Work out the finished part from the listing and answer in its coordinate system (mm). Face numbers are marked on the shaded views. A direction names the side the tool comes from. Round coordinates to 2 decimals unless told otherwise and drop trailing zeros. Write each loop counter-clockwise with the first axis right and the second up, starting at its lowest first coordinate (ties: lowest second). Pieces come first, ordered by that corner, then holes. Notation, with made-up numbers: M 39,34 L 95,34 A38 cw 95,72 Z; hole C 35.25,78.25 d6. An arc over 180 degrees is marked long. One line per item, written item: value. Start each with the question number.
Q1. Find section A-A (z = 19.15). Write down the section's boundary in (x, y), and give its area (3 significant figures).
Q2. A tool of negligible diameter and unlimited length cuts with its end or side. For the marked faces 1 and 2, from which of +Z, -Z, +X, -X, +Y, -Y can it reach the whole face along a straight path? Write none if from no direction.
Q3. Find section B-B (x = 8.5). Write down the section's boundary in (y, z), and give its area (3 significant figures).
Q4. The mould has two halves that part along X. Classify the marked faces 3, 4, 5 and 6: released by +X, released by -X, zero draft, split by the parting line, or undercut.
Q5. Consider probe 1 along Y at (x, z) = (10.75, 21.05); probe 2 along X at (y, z) = (-19, 19.85); probe 3 along Z at (x, y) = (13.75, -18.25). Determine where each line is inside the solid, lowest interval first.
Q6. Find section C-C (x = 20.25). Write down the section's boundary in (y, z), and give its area (3 significant figures).
Q7. Given pin 1 Ø3 at (x, y) = (10, -19) entering from +Z, flat-ended and moving along its own axis, determine where the tip first touches the part or whether it passes through.
from build123d import *

# Parameters (mm, degrees)
CROQUIS1_W                        = 21.8
CROQUIS1_H                        = 30
SALIENTE_EXTRUIR1_DEPTH           = 21.8
CROQUIS6_R                        = 2
CORTAR_EXTRUIR2_DEPTH             = 21.8
CORTAR_EXTRUIR4_REACH             = 45.017
CROQUIS11_R                       = 3.5
CROQUIS11_W                       = 3.4
CROQUIS11_H                       = 8.4
CORTAR_EXTRUIR4_DIRECTION_2_DEPTH = 3.5
REDONDEO1_R                       = 5
CROQUIS13_R                       = 3.5
CORTAR_EXTRUIR6_DEPTH             = 3.5
CROQUIS16_W                       = 10.1
CROQUIS16_H                       = 20.1
CORTAR_EXTRUIR7_DEPTH             = 2
CROQUIS17_W                       = 10.1
CROQUIS17_H                       = 20.1
CORTAR_EXTRUIR8_DEPTH             = 2.1
CORTAR_EXTRUIR9_START             = -3.5
CROQUIS7_R                        = 3.5
CORTAR_EXTRUIR9_DEPTH             = 3.5
CORTAR_EXTRUIR10_REACH            = 45.017
CROQUIS18_W                       = 18.8
CROQUIS18_H                       = 30


with BuildPart() as part:
    # Croquis1 → Saliente-Extruir1 (new body)
    with BuildSketch(Plane(origin=(0, 0, 0), x_dir=(0, 0, -1), z_dir=(1, 0, 0))):
        with Locations((-10.9, -15)):
            Rectangle(CROQUIS1_W, CROQUIS1_H)
    extrude(amount=SALIENTE_EXTRUIR1_DEPTH)

    # Croquis6 → Cortar-Extruir2 (cut)
    with BuildSketch(Plane.ZY):
        with Locations((10.9, -22)):
            Circle(CROQUIS6_R)
        with Locations((10.9, -7)):
            Circle(CROQUIS6_R)
    extrude(amount=-CORTAR_EXTRUIR2_DEPTH, mode=Mode.SUBTRACT)

    # Cortar-Extruir4: up to this face of the body (flat: up to its plane)
    cortar_extruir4_end = Plane(part.part.faces().sort_by_distance((10.9, 0, 10.9))[0])
    # Croquis11 → Cortar-Extruir4 (cut, up to the picked face)
    with BuildSketch(Plane.XZ.offset(30), mode=Mode.PRIVATE) as cortar_extruir4_sk1:
        with Locations(Location((13.4, 10.9, 0), (0, 0, 270))):
            Circle(CROQUIS11_R)
    cortar_extruir4_tool1 = split(extrude(cortar_extruir4_sk1.sketch, amount=-CORTAR_EXTRUIR4_REACH, mode=Mode.PRIVATE), bisect_by=cortar_extruir4_end, keep=Keep.BOTH, mode=Mode.PRIVATE)
    # Croquis11 → Cortar-Extruir4 (cut, up to the picked face)
    with BuildSketch(Plane.XZ.offset(30), mode=Mode.PRIVATE) as cortar_extruir4_sk2:
        with Locations((7.2, 10.9)):
            Rectangle(CROQUIS11_W, CROQUIS11_H)
    cortar_extruir4_tool2 = split(extrude(cortar_extruir4_sk2.sketch, amount=-CORTAR_EXTRUIR4_REACH, mode=Mode.PRIVATE), bisect_by=cortar_extruir4_end, keep=Keep.BOTH, mode=Mode.PRIVATE)
    add(cortar_extruir4_tool1.solids().sort_by(Axis((13.4, -30, 10.9), (0, 1, 0)))[0], mode=Mode.SUBTRACT)
    add(cortar_extruir4_tool2.solids().sort_by(Axis((7.2, -30, 10.9), (0, 1, 0)))[0], mode=Mode.SUBTRACT)

    # Croquis11 → Cortar-Extruir4 direction 2 (cut)
    with BuildSketch(Plane.XZ.offset(30)):
        with Locations(Location((13.4, 10.9, 0), (0, 0, 270))):
            Circle(CROQUIS11_R)
        with Locations((7.2, 10.9)):
            Rectangle(CROQUIS11_W, CROQUIS11_H)
    extrude(amount=CORTAR_EXTRUIR4_DIRECTION_2_DEPTH, mode=Mode.SUBTRACT)

    # Redondeo1
    # the kernel refuses this fillet: 5 mm, written as the material it takes off along each edge
    with BuildSketch(Plane(origin=(21.8, -30, 34.3), x_dir=(0, 1, 0), z_dir=(0, 0, -1)), Plane(origin=(0, 0, -12.5), x_dir=(1, 0, 0), z_dir=(0, 0, 1))) as redondeo1_piece_1:
        with BuildLine():
            CenterArc((REDONDEO1_R, -REDONDEO1_R), REDONDEO1_R, 90, 90)
            Line((0, -REDONDEO1_R), (0, 0))
            Line((0, 0), (REDONDEO1_R, 0))
        make_face()
    extrude(amount=46.8, mode=Mode.SUBTRACT)
    with BuildSketch(Plane(origin=(21.8, 0, -12.5), x_dir=(-1, 0, 0), z_dir=(0, 0, 1)), Plane(origin=(0, -30, 34.3), x_dir=(0, 1, 0), z_dir=(0, 0, -1))) as redondeo1_piece_2:
        with BuildLine():
            CenterArc((REDONDEO1_R, REDONDEO1_R), REDONDEO1_R, 180, 90)
            Line((0, REDONDEO1_R), (0, 0))
            Line((0, 0), (REDONDEO1_R, 0))
        make_face()
    extrude(amount=46.8, mode=Mode.SUBTRACT)

    # Croquis13 → Cortar-Extruir6 (cut)
    with BuildSketch(Plane.ZY):
        with Locations((10.9, -7)):
            Circle(CROQUIS13_R)
        with Locations(Location((10.9, -22, 0), (0, 0, 301.002719134))):
            Circle(CROQUIS13_R)
    extrude(amount=-CORTAR_EXTRUIR6_DEPTH, mode=Mode.SUBTRACT)

    # Croquis16 → Cortar-Extruir7 (cut)
    with BuildSketch(Plane.XY.offset(21.8)):
        with Locations((10.9, -15)):
            Rectangle(CROQUIS16_W, CROQUIS16_H)
    extrude(amount=-CORTAR_EXTRUIR7_DEPTH, mode=Mode.SUBTRACT)

    # Croquis17 → Cortar-Extruir8 (cut)
    with BuildSketch(Plane(origin=(0, 0, 0), x_dir=(-1, 0, 0), z_dir=(0, 0, -1))):
        with Locations((-10.9, -15)):
            Rectangle(CROQUIS17_W, CROQUIS17_H)
    extrude(amount=-CORTAR_EXTRUIR8_DEPTH, mode=Mode.SUBTRACT)

    # Croquis7 → Cortar-Extruir9 (cut)
    with BuildSketch(Plane(origin=(21.8, 0, 0), x_dir=(0, 0, -1), z_dir=(1, 0, 0)).offset(CORTAR_EXTRUIR9_START)):
        with Locations(Location((-10.9, -22, 0), (0, 0, 238.997280866))):
            Circle(CROQUIS7_R)
        with Locations(Location((-10.9, -7, 0), (0, 0, 180))):
            Circle(CROQUIS7_R)
    extrude(amount=CORTAR_EXTRUIR9_DEPTH, mode=Mode.SUBTRACT)

    # Cortar-Extruir10: up to this face of the body (flat: up to its plane)
    cortar_extruir10_end = Plane(part.part.faces().sort_by_distance((21.8, -14.963855914, 10.9))[0])
    # Croquis18 → Cortar-Extruir10 (cut, up to the picked face)
    with BuildSketch(Plane.ZY, mode=Mode.PRIVATE) as cortar_extruir10_sk1:
        with Locations((9.4, -15)):
            Rectangle(CROQUIS18_W, CROQUIS18_H)
    cortar_extruir10_tool1 = split(extrude(cortar_extruir10_sk1.sketch, amount=-CORTAR_EXTRUIR10_REACH, mode=Mode.PRIVATE), bisect_by=cortar_extruir10_end, keep=Keep.BOTH, mode=Mode.PRIVATE)
    add(cortar_extruir10_tool1.solids().sort_by(Axis((0, -15, 9.4), (1, 0, 0)))[0], mode=Mode.SUBTRACT)


solid = part.part
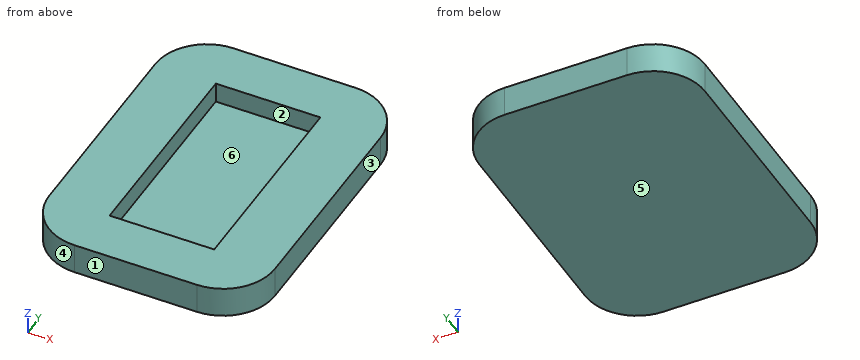
The answers:
1. outline: M 0,-25 A5 ccw 5,-30 L 16.8,-30 A5 ccw 21.8,-25 L 21.8,-5 A5 ccw 16.8,0 L 5,0 A5 ccw 0,-5 Z
1. area: 633 mm2
2. face 1: +Z, -Z, +X, -X, -Y
2. face 2: +Z
3. outline: M -30,18.8 L 0,18.8 L 0,21.8 L -4.95,21.8 L -4.95,19.8 L -25.05,19.8 L -25.05,21.8 L -30,21.8 Z
3. area: 49.8 mm2
4. face 3: released by +X
4. face 4: released by -X
4. face 5: zero draft
4. face 6: undercut
5. probe 1: -30 to -25.05, -4.95 to 0
5. probe 2: 0 to 5.85, 15.95 to 21.8
5. probe 3: 18.8 to 19.8
6. outline: M -28.62,18.8 L -1.38,18.8 L -1.38,21.8 L -28.62,21.8 Z
6. area: 81.7 mm2
7. pin 1: z = 19.8
